```python
from build123d import *

# Parameters (mm, degrees)
F1_DEPTH = 10
F3_DEPTH = 18.3104010768
F5_DEPTH = 35.001
F6_W     = 10
F6_H     = 8.9491856137
F6_R     = 3
F7_DEPTH = 2


# Not quite as in the source:
# - a pattern or mirror of a feature is missing from the dataset's text; its kind, count and spacing are read off the source's solid


with BuildPart() as f1:
    # F0 (on Front) → F1 (new body, symmetric)
    with BuildSketch(Plane.XZ):
        with BuildLine():
            Line((-3.7527767497, 1.5), (-3.4641016043, 2.0000000188))
            Line((-3.4641016043, 2.0000000188), (0, 8))
            Line((0, 8), (0, 17.5))
            Line((0, 17.5), (-18.3094010768, 17.5))
            Line((-18.3094010768, 17.5), (-18.3094010768, 8))
            Line((-18.3094010768, 8), (-14.556624327, 1.5))
            ThreePointArc((-14.556624327, 1.5), (-14.1547005384, 0), (-14.556624327, -1.5))
            Line((-14.556624327, -1.5), (-18.3094010768, -8))
            Line((-18.3094010768, -8), (-18.3094010768, -17.5))
            Line((-18.3094010768, -17.5), (0, -17.5))
            Line((0, -17.5), (0, -8))
            Line((0, -8), (-3.4641016187, -1.9999999939))
            Line((-3.4641016187, -1.9999999939), (-3.7527767497, -1.5))
            ThreePointArc((-3.7527767497, -1.5), (-4.1547005384, 0), (-3.7527767497, 1.5))
        make_face()
    extrude(amount=F1_DEPTH, both=True)

    # F2 (on Right) → F3 (cut, through all)
    with BuildSketch(Plane.YZ):
        with BuildLine():
            ThreePointArc((-6.7017059222, 0), (-7.2468927023, 4.1411047244), (-8.8452994645, 8.0000000049))
            Line((-8.8452994645, 8), (-10, 8))
            Line((-10, 8), (-10, 1.5))
            Line((-10, 1.5), (-10, -8))
            Line((-10, -8), (-10, -9.7296796796))
            ThreePointArc((-10, -9.7296796796), (-9.3945168749, -8.8836208643), (-8.8452995254, -8.0000001104))
            ThreePointArc((-8.8452995254, -8.0000001104), (-7.246892718, -4.1411047832), (-6.7017059222, 0))
        make_face()
        with BuildLine():
            ThreePointArc((-8.8452994645, 8.0000000049), (-9.3945168411, 8.8836208136), (-10, 9.7296796796))
            Line((-10, 9.7296796796), (-10, 8))
            Line((-10, 8), (-8.8452994645, 8))
        make_face()
        with BuildLine():
            Line((-5.6698729811, 2.5), (-8.8452994645, 8.0000000049))
            ThreePointArc((-8.8452994645, 8.0000000049), (-7.2468927023, 4.1411047244), (-6.7017059222, 0))
            ThreePointArc((-6.7017059222, 0), (-7.246892718, -4.1411047832), (-8.8452995254, -8.0000001104))
            Line((-8.8452995254, -8.0000001104), (-5.6698729811, -2.5))
            ThreePointArc((-5.6698729811, -2.5), (-5, 0), (-5.6698729811, 2.5))
        make_face()
        with BuildLine():
            Line((-8.8452994645, 8.0000000049), (-10, 10))
            Line((-10, 10), (-10, 9.7296796796))
            ThreePointArc((-10, 9.7296796796), (-9.3945168411, 8.8836208136), (-8.8452994645, 8.0000000049))
        make_face()
        with BuildLine():
            ThreePointArc((-8.8452995254, -8.0000001104), (-9.3945168749, -8.8836208643), (-10, -9.7296796796))
            Line((-10, -9.7296796796), (-10, -10))
            Line((-10, -10), (-8.8452995254, -8.0000001104))
        make_face()
    f3 = extrude(amount=-F3_DEPTH, mode=Mode.SUBTRACT)

    # F3_copies: F3 across plane
    add(f3.mirror(Plane.ZX), mode=Mode.SUBTRACT)

    # F4 (on face) → F5 (cut, through all)
    with BuildSketch(Plane(origin=(0, 0, -17.5), x_dir=(1, 0, 0), z_dir=(0, 0, -1))):
        with BuildLine():
            Line((-11.1804351675, 2.2127808776), (-7.1289659092, -2.2127808776))
            ThreePointArc((-7.1289659092, -2.2127808776), (-6.4090490777, -1.2088829787), (-6.1547005384, 0))
            ThreePointArc((-6.1547005384, 0), (-7.9458175596, 2.7456514607), (-11.1804351675, 2.2127808776))
        make_face()
        with BuildLine():
            ThreePointArc((-11.1804351675, 2.2127808776), (-11.367481416, -2.0257346291), (-7.1289659092, -2.2127808776))
            Line((-7.1289659092, -2.2127808776), (-11.1804351675, 2.2127808776))
        make_face()
    extrude(amount=-F5_DEPTH, mode=Mode.SUBTRACT)

    # F6 (on face) → F7 (join)
    with BuildSketch(Plane.XY.offset(17.5)):
        with Locations((-9.1547005384, 0)):
            Rectangle(F6_W, F6_H)
        with Locations((-9.1547005384, 0)):
            Circle(F6_R, mode=Mode.SUBTRACT)
    extrude(amount=F7_DEPTH)


solid = f1.part
```
Geometry check sheet. Reference: the model listing, model coordinates, mm. A direction names the side the tool comes from. Coordinates: 2 decimals unless noted, no trailing zeros. Order: outer loops, then holes, each group sorted by start corner. A loop starts at its lowest first (then second) coordinate and runs counter-clockwise, first axis right, second up.
Item 1: Depth check by flat-ended pin: pin 1 (0.6 mm diameter, centred on y = 0.5, z = 19, fed in from -X); pin 2 (10 mm diameter, centred on x = -10, z = 3.5, fed in from +Y); pin 3 (0.6 mm diameter, centred on x = -7, z = 19, fed in from -Y). Enter the tip coordinate at first touch or a pass-through.
Item 2: Scan lines: line 1 along X through (y, z) = (0, 18.4); line 2 along X through (y, z) = (-2.75, 9.5); line 3 along Y through (x, z) = (-11.5, -13). Record each from-to range of solid material in increasing order.
Item 3: Section check B-B (y = 3.75). Enter the section's corners in (x, z), plus the area to 3 significant figures.
Item 4: Section check C-C (x = -16). Enter the section's corners in (y, z).
Item 5: Tool access check on faces 1 (the flat face through (-14.155, 0, 18)), 2 (the flat face through (-16.407, -0.124, -4.705)), 3 (the flat face through (-9, -4.475, 18)), 4 (the flat face through (-4.155, 0, 18)). Record the directions out of +Z, -Z, +X, -X, +Y, -Y that give a thin tool (end or side, any length) a straight path to the whole face; none if there is none.
Item 6: Section check D-D (y = -8). Enter the section's corners in (x, z).
Item 7: Section check A-A (z = -13.5). Enter the section's corners in (x, y), plus the area to 3 significant figures.
Check sheet entries:
1. pin 1: stops at x = -14.15
1. pin 2: stops at y = 9.13
1. pin 3: stops at y = -4.47
2. line 1: x = -14.15 to -12.15, -6.15 to -4.15
2. line 2: x = -18.31 to -10.35, -7.96 to 0
2. line 3: y = -10 to -1.87, 1.87 to 10
3. outline: (-18.31, -17.5) - (0, -17.5) - (0, -8) - (-3.75, -1.5) arc R3 cw to (-3.75, 1.5) - (0, 8) - (0, 17.5) - (-4.15, 17.5) - (-4.15, 19.5) - (-14.15, 19.5) - (-14.15, 17.5) - (-18.31, 17.5) - (-18.31, 8) - (-14.56, 1.5) arc R3 cw to (-14.56, -1.5) - (-18.31, -8) - close
3. area: 588 mm2
4. outline: (-10, -17.5) - (10, -17.5) - (10, -10) - (6.54, -4) - (-6.54, -4) - (-10, -10) - close; (-10, 10) - (-6.54, 4) - (6.54, 4) - (10, 10) - (10, 17.5) - (-10, 17.5) - close
5. face 1: +Z, -X, +Y, -Y
5. face 2: -X, +Y, -Y
5. face 3: +Z, +X, -X, -Y
5. face 4: +Z, +X, +Y, -Y
6. outline: (-18.31, -17.5) - (0, -17.5) - (0, -8) - (-0.85, -6.54) - (-17.46, -6.54) - (-18.31, -8) - close; (-18.31, 8) - (-17.46, 6.54) - (-0.85, 6.54) - (0, 8) - (0, 17.5) - (-18.31, 17.5) - close
7. outline: (-18.31, -10) - (0, -10) - (0, 10) - (-18.31, 10) - close; hole circle Ø6 at (-9.15, 0)
7. area: 338 mm2
